from build123d import *

# Parameters (mm, degrees)
FILLET1_R = 2
FILLET2_R = 3


with BuildPart() as part:
    # Sketch1 → Revolve1 (revolve)
    with BuildSketch(Plane.XY, mode=Mode.PRIVATE) as revolve1_sk:
        Polygon((0, 0), (0, 154.2), (22.2, 154.2), (22.4, 110.3), (24.8, 110.3), (24.8, 107.63), (24.95, 107.63), (24.95, 93.26), (22.25, 93.26), (22.25, 85.09), (21.75, 85.09), (21.75, 0), align=None)
    revolve(revolve1_sk.sketch.rotate(Axis((0, 0, 0), (0, 1, 0)), 90), axis=Axis((0, 0, 0), (0, 1, 0)))

    # Fillet1
    fillet1_edges = [part.edges().sort_by_distance(p)[0] for p in [
        (0, 154.2, 22.2),
    ]]
    fillet(fillet1_edges, radius=FILLET1_R)

    # Fillet2
    fillet2_edges = [part.edges().sort_by_distance(p)[0] for p in [
        (0, 0, 21.75),
    ]]
    fillet(fillet2_edges, radius=FILLET2_R)


solid = part.part
For this review, take the finished solid that the model builds, in its own axes (mm). A direction names the side the tool comes from. Round coordinates to 2 decimals unless told otherwise and drop trailing zeros. Write each loop counter-clockwise with the first axis right and the second up, starting at its lowest first coordinate (ties: lowest second). Pieces come first, ordered by that corner, then holes. Notation, with made-up numbers: (42, -11.75) -> (60, -11.75) arc R27 ccw to (60, 5.25) -> close; hole circle Ø7 at (13, -36). An arc over 180 degrees is marked (long way). Put each result on its own line as item: value.
Q1. Clearance check with flat-ended pins moving along their axes: pin 1 Ø2 at (y, z) = (62.5, 6) entering from +X; pin 2 Ø1 at (x, y) = (-6.5, 53) entering from +Z; pin 3 Ø8 at (y, z) = (35.5, 16) entering from +X; pin 4 Ø13.5 at (x, z) = (8.5, -10.5) entering from -Y. State where each tip first meets the part, or that it passes through.
Determined:
pin 1: stops at x = 21.17
pin 2: stops at z = 20.91
pin 3: stops at x = 18.14
pin 4: stops at y = 0
Q2. Machinability: for faces 1 (the cylindrical face through (-21.565, 43.47, 2.831)), 2 (the flat face through (0, 0, 0)), 3 (the cylindrical face through (-7.449, 108.946, -23.655)), which of the approach directions +Z, -Z, +X, -X, +Y, -Y give a long, thin tool a straight path to every point of the face, cutting with its end or side? Answer none if there is none.
Determined:
face 1: -Y
face 2: +Z, -Z, +X, -X, -Y
face 3: +Y
Q3. Consider section A-A on y = 54.5. State the section outline as (x, z) points.
Determined:
outline: circle Ø43.5 at (0, 0)
Q4. To check wall thickness, follow L1, parallel to Y at x = 11.5, z = -20.5; L2, parallel to X at y = 88, z = -18; L3, parallel to X at y = 68.5, z = -2. State the ranges of each line that lie inside material, in increasing order. Write a range as [from, to].
Determined:
L1: y = [93.26, 110.3]
L2: x = [-13.08, 13.08]
L3: x = [-21.66, 21.66]
Q5. Consider section B-B on y = 138. State the section outline as (x, z) points, and give its area (3 significant figures).
Determined:
outline: circle Ø44.55 at (0, 0)
area: 1,560 mm^2
